Part model, mm, in its own coordinate system. A direction names the side the tool comes from. Round coordinates to 2 decimals unless told otherwise and drop trailing zeros. Order: outer loops, then holes, each group sorted by start corner. A loop starts at its lowest first (then second) coordinate and runs counter-clockwise, first axis right, second up. Notation, with made-up numbers: (61, 3.25) - (101, 3.25) arc R29 ccw to (101, 25.25) - close; hole circle Ø3 at (-8, -39). An arc over 180 degrees is marked (long way). Answer as a JSON object with one key per item and string values.
```python
from build123d import *
from build123d.topology import SkipClean

# Parameters (mm, degrees)
SKETCH1_W           = 120
SKETCH1_H           = 52.5
BOSS_EXTRUDE1_DEPTH = 6
CUT_EXTRUDE1_DEPTH  = 6
SKETCH3_W           = 23
SKETCH3_H           = 4
CUT_EXTRUDE2_DEPTH  = 6
SKETCH4_W           = 42.25
SKETCH4_H           = 21.5
CUT_EXTRUDE3_DEPTH  = 6
SKETCH5_W           = 8
SKETCH5_H           = 21.5
SKETCH5_W_2         = 15.5
CUT_EXTRUDE4_DEPTH  = 3
SKETCH6_W           = 17
SKETCH6_H           = 72.5
BOSS_EXTRUDE2_DEPTH = 12
CUT_EXTRUDE6_DEPTH  = 136.831697332
SKETCH8_W           = 17
SKETCH8_H           = 36.25
CUT_EXTRUDE7_DEPTH  = 137.492673796
SKETCH9_W           = 65.75
SKETCH9_H           = 10.75
CUT_EXTRUDE8_DEPTH  = 6
SKETCH10_W          = 5
SKETCH10_H          = 6
BOSS_EXTRUDE3_DEPTH = 10
SKETCH14_R          = 2
CUT_EXTRUDE9_DEPTH  = 3
SKETCH15_R          = 2.25
CUT_EXTRUDE10_DEPTH = 136.831697332
SKETCH17_R          = 2
CUT_EXTRUDE11_DEPTH = 136.831697332
SKETCH18_W          = 11
SKETCH18_H          = 20.25
CUT_EXTRUDE12_DEPTH = 12
SKETCH19_R          = 1.75
CUT_EXTRUDE13_DEPTH = 132.248809518
SKETCH20_W          = 11
SKETCH20_H          = 16
CUT_EXTRUDE14_DEPTH = 6
SKETCH21_W          = 63
SKETCH21_H          = 6
BOSS_EXTRUDE6_DEPTH = 6
SKETCH22_W          = 6
SKETCH22_H          = 40.5
BOSS_EXTRUDE7_DEPTH = 6
BOSS_EXTRUDE8_START = 6
SKETCH24_R          = 2.25
BOSS_EXTRUDE8_DEPTH = 6


with BuildPart() as part:
    # Sketch1 → Boss-Extrude1 (new body)
    with BuildSketch(Plane(origin=(0, 0, 0), x_dir=(1, 0, 0), z_dir=(0, 1, 0))):
        with Locations((60, 26.25)):
            Rectangle(SKETCH1_W, SKETCH1_H)
    extrude(amount=BOSS_EXTRUDE1_DEPTH)

    # Sketch2 → Cut-Extrude1 (cut)
    with BuildSketch(Plane(origin=(0, 6, 0), x_dir=(1, 0, 0), z_dir=(0, 1, 0))):
        Polygon((0, 0), (16, 0), (0, 5.25), align=None)
        Polygon((0, 47.25), (0, 52.5), (16, 52.5), align=None)
    extrude(amount=-CUT_EXTRUDE1_DEPTH, mode=Mode.SUBTRACT)

    # Sketch3 → Cut-Extrude2 (cut)
    with BuildSketch(Plane(origin=(0, 6, 0), x_dir=(1, 0, 0), z_dir=(0, 1, 0))):
        with Locations((28.5, 2)):
            Rectangle(SKETCH3_W, SKETCH3_H)
        with Locations((28.5, 50.5)):
            Rectangle(SKETCH3_W, SKETCH3_H)
    extrude(amount=-CUT_EXTRUDE2_DEPTH, mode=Mode.SUBTRACT)

    # Sketch4 → Cut-Extrude3 (cut)
    with BuildSketch(Plane(origin=(0, 6, 0), x_dir=(1, 0, 0), z_dir=(0, 1, 0))):
        with Locations((40.625, 26.25)):
            Rectangle(SKETCH4_W, SKETCH4_H)
    extrude(amount=-CUT_EXTRUDE3_DEPTH, mode=Mode.SUBTRACT)

    # Sketch5 → Cut-Extrude4 (cut)
    with BuildSketch(Plane(origin=(0, 6, 0), x_dir=(1, 0, 0), z_dir=(0, 1, 0))):
        with Locations((65.75, 26.25)):
            Rectangle(SKETCH5_W, SKETCH5_H)
        with Locations((11.75, 26.25)):
            Rectangle(SKETCH5_W_2, SKETCH5_H)
    extrude(amount=-CUT_EXTRUDE4_DEPTH, mode=Mode.SUBTRACT)

    # Sketch6 → Boss-Extrude2 (add)
    with BuildSketch(Plane(origin=(0, 6, 0), x_dir=(1, 0, 0), z_dir=(0, 1, 0))):
        with Locations((111.5, 26.25)):
            Rectangle(SKETCH6_W, SKETCH6_H)
    extrude(amount=BOSS_EXTRUDE2_DEPTH)

    # Sketch7 → Cut-Extrude6 (cut, through all)
    with BuildSketch(Plane(origin=(0, 6, 0), x_dir=(1, 0, 0), z_dir=(0, 1, 0))):
        Polygon((103, 26.25), (69.75, 26.25), (69.75, 15.5), (4, 15.5), (4, 26.25), (0, 26.25), (0, 5.25), (16, 0), (17, 0), (17, 4), (40, 4), (40, 0), (103, 0), align=None)
    extrude(amount=-CUT_EXTRUDE6_DEPTH, mode=Mode.SUBTRACT)

    # Sketch8 → Cut-Extrude7 (cut, through all)
    with BuildSketch(Plane(origin=(0, 18, 0), x_dir=(1, 0, 0), z_dir=(0, 1, 0))):
        with Locations((111.5, 8.125)):
            Rectangle(SKETCH8_W, SKETCH8_H)
    extrude(amount=-CUT_EXTRUDE7_DEPTH, mode=Mode.SUBTRACT)

    # Sketch9 → Cut-Extrude8 (cut)
    with BuildSketch(Plane(origin=(0, 3, 0), x_dir=(1, 0, 0), z_dir=(0, 1, 0))):
        with Locations((36.875, 20.875)):
            Rectangle(SKETCH9_W, SKETCH9_H)
    extrude(amount=-CUT_EXTRUDE8_DEPTH, mode=Mode.SUBTRACT)

    # Sketch10 → Boss-Extrude3 (add)
    with BuildSketch(Plane(origin=(0, 0, -52.5), x_dir=(-1, 0, 0), z_dir=(0, 0, -1))):
        with Locations((-117.5, 3)):
            Rectangle(SKETCH10_W, SKETCH10_H)
    extrude(amount=BOSS_EXTRUDE3_DEPTH)

    # Sketch14 → Cut-Extrude9 (cut)
    with BuildSketch(Plane(origin=(0, 3, 0), x_dir=(1, 0, 0), z_dir=(0, 1, 0))):
        with Locations(Location((66, 30.75, 0), (0, 0, 270))):
            Circle(SKETCH14_R)
        with Locations(Location((15.25, 30.75, 0), (0, 0, 270))):
            Circle(SKETCH14_R)
    extrude(amount=-CUT_EXTRUDE9_DEPTH, mode=Mode.SUBTRACT)

    # Sketch15 → Cut-Extrude10 (cut, through all)
    with BuildSketch(Plane(origin=(0, 6, 0), x_dir=(1, 0, 0), z_dir=(0, 1, 0))):
        with Locations(Location((6, 43.25, 0), (0, 0, 270))):
            Circle(SKETCH15_R)
    extrude(amount=-CUT_EXTRUDE10_DEPTH, mode=Mode.SUBTRACT)

    # Sketch17 → Cut-Extrude11 (cut, through all)
    with BuildSketch(Plane.XZ.offset(-6)):
        with Locations(Location((109, -57.5, 0), (0, 0, 270))):
            Circle(SKETCH17_R)
    extrude(amount=-CUT_EXTRUDE11_DEPTH, mode=Mode.SUBTRACT)

    # Sketch18 → Cut-Extrude12 (cut)
    with BuildSketch(Plane(origin=(0, 18, 0), x_dir=(1, 0, 0), z_dir=(0, 1, 0))):
        with Locations((108.5, 36.375)):
            Rectangle(SKETCH18_W, SKETCH18_H)
    extrude(amount=-CUT_EXTRUDE12_DEPTH, mode=Mode.SUBTRACT)

    # Sketch19 → Cut-Extrude13 (cut, through all)
    with BuildSketch(Plane.ZY.offset(-114)):
        with Locations((-41.25, 12)):
            Circle(SKETCH19_R)
        with Locations((-26.25, 12)):
            Circle(SKETCH19_R)
    extrude(amount=-CUT_EXTRUDE13_DEPTH, mode=Mode.SUBTRACT)

    # Sketch20 → Cut-Extrude14 (cut)
    with BuildSketch(Plane(origin=(0, 18, 0), x_dir=(1, 0, 0), z_dir=(0, 1, 0))):
        with Locations((108.5, 54.5)):
            Rectangle(SKETCH20_W, SKETCH20_H)
    extrude(amount=-CUT_EXTRUDE14_DEPTH, mode=Mode.SUBTRACT)

    # Sketch21 → Boss-Extrude6 (add)
    with BuildSketch(Plane(origin=(0, 6, 0), x_dir=(1, 0, 0), z_dir=(0, 1, 0))):
        with Locations((71.5, 49.5)):
            Rectangle(SKETCH21_W, SKETCH21_H)
    extrude(amount=BOSS_EXTRUDE6_DEPTH)

    # Mirror1: part across plane


with BuildPart() as part_1:
    with SkipClean():  # the faces are left unmerged after this step: merging them gives an invalid solid
        add(part.part)
        add(part.part.mirror(Plane(origin=(103, -2.5e-05, -26.25), x_dir=(1, 0, 0), z_dir=(0, 0, -1))))

    # Sketch22 → Boss-Extrude7 (add)
    with SkipClean():  # the faces are left unmerged after this step: merging them gives an invalid solid
        with BuildSketch(Plane(origin=(0, 6, 0), x_dir=(1, 0, 0), z_dir=(0, 1, 0))):
            with Locations((82.75, 26.25)):
                Rectangle(SKETCH22_W, SKETCH22_H)
            with Locations((98.75, 26.25)):
                Rectangle(SKETCH22_W, SKETCH22_H)
        extrude(amount=BOSS_EXTRUDE7_DEPTH)

    # Sketch24 → Boss-Extrude8 (add)
    with BuildSketch(Plane(origin=(0, 6, 0), x_dir=(1, 0, 0), z_dir=(0, 1, 0)).offset(BOSS_EXTRUDE8_START)):
        Polygon((17, 15.5), (17, 0), (16, 0), (0, 5.25), (0, 47.25), (16, 52.5), (17, 52.5), (17, 37), (4, 37), (4, 15.5), align=None)
        with Locations(Location((6, 43.25, 0), (0, 0, 270))):
            Circle(SKETCH24_R, mode=Mode.SUBTRACT)
        with Locations(Location((6, 9.25, 0), (0, 0, 90))):
            Circle(SKETCH24_R, mode=Mode.SUBTRACT)
    extrude(amount=-BOSS_EXTRUDE8_DEPTH)


solid = part_1.part
```
Item 1: Tool access for faces 1 (the flat face through (0, 6, -26)), 2 (the flat face through (40, 6, -2)), 3 (the flat face through (85, 12, -29)), 4 (the flat face through (19.5, 2, -26)), 5 (the flat face through (69.75, 5, -26)): list every direction of +Z, -Z, +X, -X, +Y, -Y with a clear straight run to the whole face (end or side of a thin tool).
Taken from the geometry:
{"face 1": "+Z, -Z, -X, +Y, -Y", "face 2": "+Z, +Y", "face 3": "+Z, -Z, -X, +Y", "face 4": "+Y, -Y", "face 5": "+Y"}
Item 2: Probe L1, parallel to X at y = 1.6, z = -30.75; L2, parallel to X at y = 7, z = -43.25; L3, parallel to Z at x = 72.5, y = 10. List the from-to ranges inside material, lowest first. Write a range as from..to.
Taken from the geometry:
{"L1": "0..13.25, 17.25..19.5, 61.75..64, 68..120", "L2": "0..3.75, 8.25..17, 79.75..85.75, 95.75..101.75, 114..120", "L3": "-52.5..-46.5, -6..0"}
Item 3: Cut at D-D (x = 58.5). Write the cut outline in (y, z), plus the area to 3 significant figures.
Taken from the geometry:
{"outline": "(0, -52.5) - (12, -52.5) - (12, -46.5) - (6, -46.5) - (6, -37) - (0, -37) - close; (0, -15.5) - (6, -15.5) - (6, -6) - (12, -6) - (12, 0) - (0, 0) - close", "area": "258 mm2"}
Item 4: Cut at A-A (z = -21.75). State how many separate pieces and enclosed holes the cut face has, plus the area to 3 significant figures.
Taken from the geometry:
{"separate pieces": "4", "enclosed holes": "0", "area": "540 mm2"}
Item 5: Two-plate mould, pull along X, no slides. Class faces 6 (the flat face through (114, 15, -27)), 7 (the flat face through (108.9, 6, 7.3)), 8 (the flat face through (103, 9, 5)), 9 (the flat face through (66, 3, -26)): pulls with the +X half, pulls with the -X half, needs draft (parallel to the pull), parting line crosses it, or undercut.
Taken from the geometry:
{"face 6": "undercut", "face 7": "needs draft", "face 8": "pulls with the -X half", "face 9": "undercut"}
Item 6: Drop flat-ended pins along their axis: P1, Ø10, axis at x = 50.5, y = 2.5, coming from the +Z side; P2, Ø4, axis at x = 32, y = 4, coming from the -Z side; P3, Ø6, axis at x = 106, z = -30.5, coming from the +Y side. Give the stop position or say it passes through.
Taken from the geometry:
{"P1": "z = 0", "P2": "z = -48.5", "P3": "y = 6"}
Item 7: Cut at B-B (x = 109). Write the cut outline in (y, z), plus the area to 3 significant figures.
Taken from the geometry:
{"outline": "(0, -52.5) - (6, -52.5) - (6, -55.5) - (12, -55.5) - (12, -46.5) - (6, -46.5) - (6, -6) - (12, -6) - (12, 3) - (6, 3) - (6, 0) - (0, 0) - close; (6, -62.5) - (12, -62.5) - (12, -59.5) - (6, -59.5) - close; (6, 7) - (12, 7) - (12, 10) - (6, 10) - close", "area": "459 mm2"}
Item 8: Cut at C-C (z = 5). Write the cut outline in (x, y).
Taken from the geometry:
{"outline": "(103, 6) - (107, 6) - (107, 12) - (103, 12) - close; (111, 6) - (115, 6) - (115, 0) - (120, 0) - (120, 18) - (114, 18) - (114, 12) - (111, 12) - close"}
